from build123d import *

# Parameters (mm, degrees)
MODEL_R                 = 1.5
SALIENTE_EXTRUIR1_DEPTH = 3


with BuildPart() as part:
    # Model → Saliente-Extruir1 (new body)
    with BuildSketch(Plane.XY):
        with BuildLine():
            Line((404.929131311, 485.242243614), (404.929131311, 404.242243614))
            ThreePointArc((404.929131311, 404.242243614), (403.611111826, 401.060263099), (400.429131311, 399.742243614))
            Line((400.429131311, 399.742243614), (256.429131311, 399.742243614))
            ThreePointArc((256.429131311, 399.742243614), (253.247150795, 401.060263099), (251.929131311, 404.242243614))
            Line((251.929131311, 404.242243614), (251.929131311, 485.242243614))
            ThreePointArc((251.929131311, 485.242243614), (253.247150795, 488.424224129), (256.429131311, 489.742243614))
            Line((256.429131311, 489.742243614), (400.429131311, 489.742243614))
            ThreePointArc((400.429131311, 489.742243614), (403.611111826, 488.424224129), (404.929131311, 485.242243614))
        make_face()
        with Locations((400.429131311, 485.242243614)):
            Circle(MODEL_R, mode=Mode.SUBTRACT)
        with Locations((400.429131311, 476.242243614)):
            Circle(MODEL_R, mode=Mode.SUBTRACT)
        with Locations((400.429131311, 467.242243614)):
            Circle(MODEL_R, mode=Mode.SUBTRACT)
        with Locations((400.429131311, 458.242243614)):
            Circle(MODEL_R, mode=Mode.SUBTRACT)
        with Locations((400.429131311, 449.242243614)):
            Circle(MODEL_R, mode=Mode.SUBTRACT)
        with Locations((400.429131311, 440.242243614)):
            Circle(MODEL_R, mode=Mode.SUBTRACT)
        with Locations((400.429131311, 431.242243614)):
            Circle(MODEL_R, mode=Mode.SUBTRACT)
        with Locations((400.429131311, 422.242243614)):
            Circle(MODEL_R, mode=Mode.SUBTRACT)
        with Locations((400.429131311, 413.242243614)):
            Circle(MODEL_R, mode=Mode.SUBTRACT)
        with Locations((400.429131311, 404.242243614)):
            Circle(MODEL_R, mode=Mode.SUBTRACT)
        with Locations((256.429131311, 485.242243614)):
            Circle(MODEL_R, mode=Mode.SUBTRACT)
        with Locations((256.429131311, 476.242243614)):
            Circle(MODEL_R, mode=Mode.SUBTRACT)
        with Locations((256.429131311, 467.242243614)):
            Circle(MODEL_R, mode=Mode.SUBTRACT)
        with Locations((256.429131311, 458.242243614)):
            Circle(MODEL_R, mode=Mode.SUBTRACT)
        with Locations((256.429131311, 449.242243614)):
            Circle(MODEL_R, mode=Mode.SUBTRACT)
        with Locations((256.429131311, 440.242243614)):
            Circle(MODEL_R, mode=Mode.SUBTRACT)
        with Locations((256.429131311, 431.242243614)):
            Circle(MODEL_R, mode=Mode.SUBTRACT)
        with Locations((256.429131311, 422.242243614)):
            Circle(MODEL_R, mode=Mode.SUBTRACT)
        with Locations((256.429131311, 413.242243614)):
            Circle(MODEL_R, mode=Mode.SUBTRACT)
        with Locations((256.429131311, 404.242243614)):
            Circle(MODEL_R, mode=Mode.SUBTRACT)
        with Locations((265.429131311, 485.242243614)):
            Circle(MODEL_R, mode=Mode.SUBTRACT)
        with Locations((265.429131311, 404.242243614)):
            Circle(MODEL_R, mode=Mode.SUBTRACT)
        with Locations((274.429131311, 485.242243614)):
            Circle(MODEL_R, mode=Mode.SUBTRACT)
        with Locations((274.429131311, 404.242243614)):
            Circle(MODEL_R, mode=Mode.SUBTRACT)
        with Locations((283.429131311, 485.242243614)):
            Circle(MODEL_R, mode=Mode.SUBTRACT)
        with Locations((283.429131311, 404.242243614)):
            Circle(MODEL_R, mode=Mode.SUBTRACT)
        with Locations((292.429131311, 485.242243614)):
            Circle(MODEL_R, mode=Mode.SUBTRACT)
        with Locations((292.429131311, 404.242243614)):
            Circle(MODEL_R, mode=Mode.SUBTRACT)
        with Locations((301.429131311, 485.242243614)):
            Circle(MODEL_R, mode=Mode.SUBTRACT)
        with Locations((301.429131311, 404.242243614)):
            Circle(MODEL_R, mode=Mode.SUBTRACT)
        with Locations((310.429131311, 485.242243614)):
            Circle(MODEL_R, mode=Mode.SUBTRACT)
        with Locations((310.429131311, 404.242243614)):
            Circle(MODEL_R, mode=Mode.SUBTRACT)
        with Locations((319.429131311, 485.242243614)):
            Circle(MODEL_R, mode=Mode.SUBTRACT)
        with Locations((319.429131311, 404.242243614)):
            Circle(MODEL_R, mode=Mode.SUBTRACT)
        with Locations((328.429131311, 485.242243614)):
            Circle(MODEL_R, mode=Mode.SUBTRACT)
        with Locations((328.429131311, 404.242243614)):
            Circle(MODEL_R, mode=Mode.SUBTRACT)
        with Locations((337.429131311, 485.242243614)):
            Circle(MODEL_R, mode=Mode.SUBTRACT)
        with Locations((337.429131311, 404.242243614)):
            Circle(MODEL_R, mode=Mode.SUBTRACT)
        with Locations((346.429131311, 485.242243614)):
            Circle(MODEL_R, mode=Mode.SUBTRACT)
        with Locations((346.429131311, 404.242243614)):
            Circle(MODEL_R, mode=Mode.SUBTRACT)
        with Locations((355.429131311, 485.242243614)):
            Circle(MODEL_R, mode=Mode.SUBTRACT)
        with Locations((355.429131311, 404.242243614)):
            Circle(MODEL_R, mode=Mode.SUBTRACT)
        with Locations((364.429131311, 485.242243614)):
            Circle(MODEL_R, mode=Mode.SUBTRACT)
        with Locations((364.429131311, 404.242243614)):
            Circle(MODEL_R, mode=Mode.SUBTRACT)
        with Locations((373.429131311, 485.242243614)):
            Circle(MODEL_R, mode=Mode.SUBTRACT)
        with Locations((373.429131311, 404.242243614)):
            Circle(MODEL_R, mode=Mode.SUBTRACT)
        with Locations((382.429131311, 485.242243614)):
            Circle(MODEL_R, mode=Mode.SUBTRACT)
        with Locations((382.429131311, 404.242243614)):
            Circle(MODEL_R, mode=Mode.SUBTRACT)
        with Locations((391.429131311, 485.242243614)):
            Circle(MODEL_R, mode=Mode.SUBTRACT)
        with Locations((391.429131311, 404.242243614)):
            Circle(MODEL_R, mode=Mode.SUBTRACT)
    extrude(amount=SALIENTE_EXTRUIR1_DEPTH)


solid = part.part
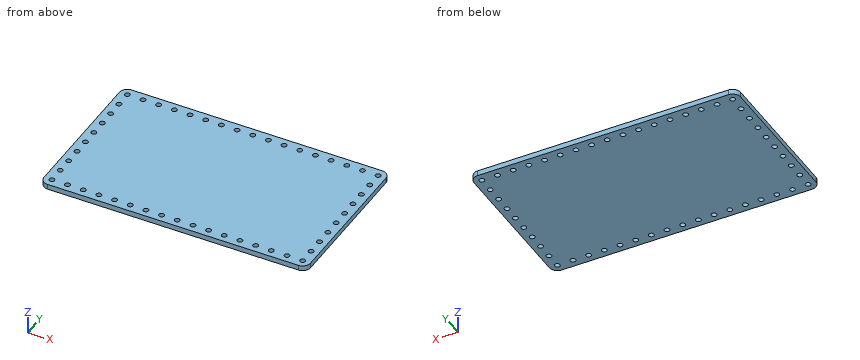
Build history of the part. All positions in model axes, mm. Give positions to 0.01 mm unless a question says otherwise; leave off trailing zeros. Use one line per item in the form item = value. Start each with the question number.
1. Drop a flat-ended pin along its axis: pin 1 Ø5 at (x, y) = (256.43, 440.24) entering from +Z. Give the stop position or say it passes through.
2. Probe line 1 (X direction, y = 458.5, z = 0.9); line 2 (Y direction, x = 329.5, z = 0.9); line 3 (X direction, y = 414, z = 2.5). List the from-to ranges inside material, lowest first. Write a range as [from, to].
3. Band-saw the part on A-A on z = 1.95. Count the separate pieces of the cut face and the enclosed holes in it, plus the area to 3 significant figures.
Conclusion:
q1.pin_1 = 3
q2.line_1 = [251.93, 254.95], [257.91, 398.95], [401.91, 404.93]
q2.line_2 = [399.74, 403.19], [405.29, 484.19], [486.29, 489.74]
q2.line_3 = [251.93, 255.13], [257.72, 399.13], [401.72, 404.93]
q3.separate_pieces = 1
q3.enclosed_holes = 50
q3.area = 13,400 mm²
